Read the model definition and answer for the solid it produces. Units are mm, in the model's axes. Coordinates: 2 decimals unless noted, no trailing zeros. Loops run counter-clockwise (first coordinate to the right, second up) from the corner with the lowest first, then second, coordinate; pieces in that order, holes last. Notation, with made-up numbers: (-22.5, 62.25) -> (13.5, 62.25) arc R31 cw to (13.5, 87.25) -> close; hole circle Ø7 at (-33.5, -10.75). An arc over 180 degrees is marked (long way). Answer as a JSON object with one key per item and string values. Group by question number.
Q1. Straight lines are drawn through the part: line 1 along Z through (x, y) = (60.5, -0.5); line 2 along X through (y, z) = (-6.5, 320.5); line 3 along Z through (x, y) = (168.5, -7.75). For each, find the intervals that lie inside material, in ascending order. Write a range as [from, to].
Q2. The part is cut by section A-A on y = -6. Write down the section's boundary in (x, z).
Q3. The part is cut by section B-B on x = 59. Write down the section's boundary in (y, z).
Q4. The part is cut by section D-D on x = 440.5. Write down the section's boundary in (y, z).
Q5. The part is cut by section C-C on z = 71. Write down the section's boundary in (x, y), and give its area (3 significant figures).
from build123d import *

# Parameters (mm, degrees)
F0_W     = 77
F0_H     = 77
F1_DEPTH = 12


with BuildPart() as f1:
    # F0 (on Front) → F1 (new body)
    with BuildSketch(Plane.XZ):
        with BuildLine():
            ThreePointArc((0, 30), (8.786797, 8.786797), (30, 0))
            Line((30, 0), (139.86896, 0))
            Line((139.86896, 0), (550, 120.816529))
            Line((550, 120.816529), (550, 320))
            ThreePointArc((550, 320), (541.213203, 341.213203), (520, 350))
            Line((520, 350), (30, 350))
            ThreePointArc((30, 350), (8.786797, 341.213203), (0, 320))
            Line((0, 320), (0, 30))
        make_face()
        with Locations((68.5, 68.5)):
            Rectangle(F0_W, F0_H, mode=Mode.SUBTRACT)
    extrude(amount=F1_DEPTH)


solid = f1.part
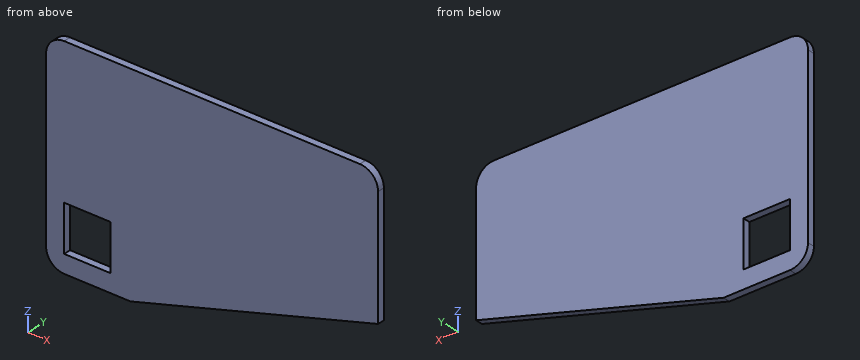
Final values:
{
 "1": {"line 1": "z = [0, 30], [107, 350]", "line 2": "x = [0, 550]", "line 3": "z = [8.43, 350]"},
 "2": {"outline": "(0, 30) arc R30 ccw to (30, 0) -> (139.87, 0) -> (550, 120.82) -> (550, 320) arc R30 ccw to (520, 350) -> (30, 350) arc R30 ccw to (0, 320) -> close; hole (30, 30) -> (107, 30) -> (107, 107) -> (30, 107) -> close"},
 "3": {"outline": "(-12, 0) -> (0, 0) -> (0, 30) -> (-12, 30) -> close; (-12, 107) -> (0, 107) -> (0, 350) -> (-12, 350) -> close"},
 "4": {"outline": "(-12, 88.56) -> (0, 88.56) -> (0, 350) -> (-12, 350) -> close"},
 "5": {"outline": "(0, -12) -> (30, -12) -> (30, 0) -> (0, 0) -> close; (107, -12) -> (380.89, -12) -> (380.89, 0) -> (107, 0) -> close", "area": "3,650 mm2"}
}
